CAD build for the part. Positions are in the model's coordinates, mm. Coordinates: 2 decimals unless noted, no trailing zeros. Order: outer loops, then holes, each group sorted by start corner. A loop starts at its lowest first (then second) coordinate and runs counter-clockwise, first axis right, second up. Notation, with made-up numbers: M -19,70 L 9,70 A25 cw 9,98 Z; hole C 61,87.25 d1. An arc over 180 degrees is marked long. Write item = value, one per line. Start each with the question number.
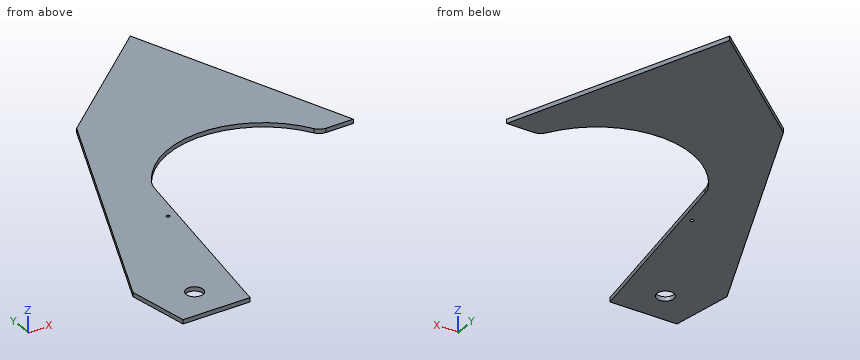
```python
from build123d import *

# Parameters (mm, degrees)
SKETCH1_R           = 6.35
BOSS_EXTRUDE1_DEPTH = 3.175
CUT_EXTRUDE3_DEPTH  = 392.229140513
FILLET1_R           = 7.62
FILLET4_R           = 25.4
SKETCH5_R           = 1.27
CUT_EXTRUDE4_DEPTH  = 392.229140513


with BuildPart() as part:
    # Sketch1 → Boss-Extrude1 (new body)
    with BuildSketch(Plane.XY):
        with BuildLine():
            Line((0, 0), (50.8, 0))
            Line((50.8, 0), (76.2, 152.4))
            ThreePointArc((76.2, 152.4), (139.7, 191.491818659), (203.2, 152.4))
            Line((203.2, 152.4), (228.6, 152.4))
            Line((228.6, 152.4), (167.642212713, 317.477872869))
            Line((167.642212713, 317.477872869), (-25.4, 152.4))
            Line((-25.4, 152.4), (0, 0))
        make_face()
        with Locations((25.4, 25.4)):
            Circle(SKETCH1_R, mode=Mode.SUBTRACT)
    extrude(amount=BOSS_EXTRUDE1_DEPTH)

    # Sketch4 → Cut-Extrude3 (cut, through all)
    with BuildSketch(Plane.XY.offset(3.175)):
        Polygon((86.239354079, 263.432711485), (-16.185204596, 26.450399258), (-107.229256751, 193.810789249), align=None)
    extrude(amount=-CUT_EXTRUDE3_DEPTH, mode=Mode.SUBTRACT)

    # Fillet1
    fillet1_edges = [part.edges().sort_by_distance(p)[0] for p in [
        (203.2, 152.4, 1.5875),
    ]]
    fillet(fillet1_edges, radius=FILLET1_R)

    # Fillet4
    fillet4_edges = [part.edges().sort_by_distance(p)[0] for p in [
        (76.2, 152.4, 1.5875),
    ]]
    fillet(fillet4_edges, radius=FILLET4_R)

    # Sketch5 → Cut-Extrude4 (cut, through all)
    with BuildSketch(Plane(origin=(0, 0, 0), x_dir=(-1, 0, 0), z_dir=(0, 0, -1))):
        with Locations((-63.412409655, 114.3)):
            Circle(SKETCH5_R)
    extrude(amount=-CUT_EXTRUDE4_DEPTH, mode=Mode.SUBTRACT)


solid = part.part
```
1. Slice it at C-C (y = 25.4). Write the cut outline in (x, z) (3 decimals), plus the area to 3 significant figures.
2. Flat gauge pin, fed straight in: pin 1 (1 mm diameter, centred on y = 157.5, z = 2.5, fed in from +X). Where does the tip first touch, or does it go through?
3. Probe L1, parallel to Y at x = 25.4, z = 0.95; L2, parallel to X at y = 114.3, z = 1.8; L3, parallel to Y at x = 21.5, z = 2.95. List the from-to ranges inside material, lowest first.
4. Slice it at B-B (x = 25.4). Write the cut outline in (y, z) (3 decimals).
5. Slice it at A-A (z = 1.45). Write the cut outline in (x, y).
6. Slice it at D-D (x = 107). Write the cut outline in (y, z) (3 decimals).
Calculated:
q1.outline = M -4.233,0 L 19.05,0 L 19.05,3.175 L -4.233,3.175 Z; M 31.75,0 L 55.033,0 L 55.033,3.175 L 31.75,3.175 Z
q1.area = 148 mm²
q2.pin_1 = 226.9
q3.L1 = 0 to 19.05, 31.75 to 122.67
q3.L2 = 21.78 to 62.14, 64.68 to 69.85
q3.L3 = 0 to 20.39, 30.41 to 113.64
q4.outline = M 0,0 L 19.05,0 L 19.05,3.175 L 0,3.175 Z; M 31.75,0 L 122.667,0 L 122.667,3.175 L 31.75,3.175 Z
q5.outline = M -7.69,46.12 L 0,0 L 50.8,0 L 75.49,148.16 A25.4 cw 78.8,157.1 A71.12 cw 201.15,156.18 A7.62 ccw 207.73,152.4 L 228.6,152.4 L 167.64,317.48 L 75.57,238.74 Z; hole C 25.4,25.4 d12.7; hole C 63.41,114.3 d2.54
q6.outline = M 183.528,0 L 265.62,0 L 265.62,3.175 L 183.528,3.175 Z
